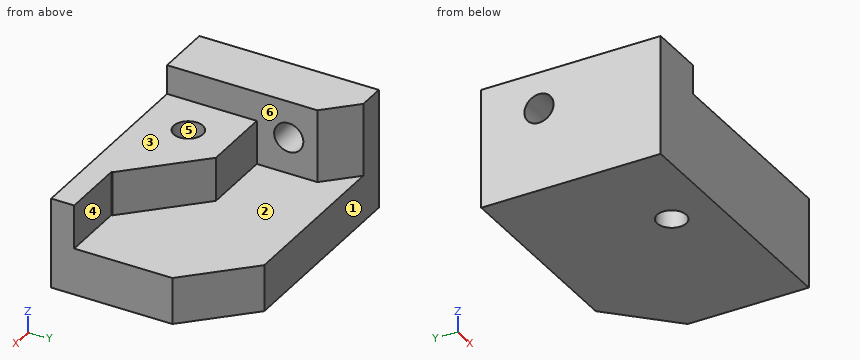
Autodesk Fusion 360 part; units mm, degrees
sketch "Sketch1" plane through (0, 0, 0) normal (0, 0, 1) x (1, 0, 0)
  line L0 (88.0885, 61.5355) -> (-88.0885, 61.5355)
  line L1 (-88.0885, 61.5355) -> (-88.0885, -61.5355)
  line L2 (-88.0885, -61.5355) -> (88.0885, -61.5355)
  line L3 (88.0885, -61.5355) -> (88.0885, 61.5355)
  line L4 (88.0885, 61.5355) -> (-88.0885, -61.5355) construction
  line L5 (-88.0885, 61.5355) -> (88.0885, -61.5355) construction
extrude "Extrude1" add sketch "Sketch1" along normal blind 32
chamfer "Chamfer1" distance 40 angle 45 1 edges at (88.0885, 61.5355, 16)
sketch "Sketch2" plane through (0, 0, 32) normal (0, 0, 1) x (-1, 0, 0)
  line L0 (-88.0885, -21.5355) -> (-48.0885, -61.5355)
  line L1 (-48.0885, -61.5355) -> (88.0885, -61.5355)
  line L2 (88.0885, -61.5355) -> (88.0885, 61.5355)
  line L3 (88.0885, 61.5355) -> (-88.0885, 61.5355)
  line L4 (-88.0885, 61.5355) -> (-88.0885, -21.5355)
  line L5 (88.0885, 61.5355) -> (49.7061, 61.5355)
  line L6 (49.7061, 61.5355) -> (49.7061, -61.5355)
  line L7 (49.7061, -61.5355) -> (88.0885, -61.5355)
  line L8 (88.0885, -61.5355) -> (88.0885, 61.5355)
extrude "Extrude2" add sketch "Sketch2" along normal blind 50 contours L1 L2 L3 L5 L6 L7 L8
sketch "Sketch3" plane through (0, 61.5355, 0) normal (0, 1, 0) x (-1, 0, 0)
  line L0 (-48.0885, 32) -> (-48.0885, 0)
  line L1 (-48.0885, 0) -> (88.0885, 0)
  line L2 (88.0885, 0) -> (88.0885, 82)
  line L3 (88.0885, 82) -> (49.7061, 82)
  line L4 (49.7061, 82) -> (49.7061, 32)
  line L5 (49.7061, 32) -> (-48.0885, 32)
chamfer "Chamfer2" distance 20 angle 45 1 edges at (-49.7061, 61.5355, 57)
sketch "Sketch4" plane through (0, 0, 32) normal (0, 0, 1) x (-1, 0, 0)
  line L0 (49.7061, -41.5355) -> (49.7061, 61.5355)
  line L1 (49.7061, 61.5355) -> (-88.0885, 61.5355)
  line L2 (-88.0885, 61.5355) -> (-88.0885, -21.5355)
  line L3 (-88.0885, -21.5355) -> (-48.0885, -61.5355)
  line L4 (-48.0885, -61.5355) -> (69.7061, -61.5355)
  line L5 (69.7061, -61.5355) -> (49.7061, -41.5355)
  line L6 (49.7061, 61.5355) -> (-43.9087, 61.5355)
  line L7 (-43.9087, 61.5355) -> (-43.9087, 0)
  line L8 (-43.9087, 0) -> (49.7061, 0)
  line L9 (49.7061, 0) -> (49.7061, 61.5355)
extrude "Extrude3" add sketch "Sketch4" along normal blind 30 contours L0 L1 L6 L7 L8 L9
chamfer "Chamfer3" distance 45 angle 45 1 edges at (43.9087, 0, 47)
sketch "Sketch5" plane through (0, 0, 32) normal (0, 0, 1) x (-1, 0, 0)
  line L0 (49.7061, 0) -> (1.0913, 0)
  line L1 (1.0913, 0) -> (-43.9087, 45)
  line L2 (-43.9087, 45) -> (-43.9087, 61.5355)
  line L3 (-43.9087, 61.5355) -> (-88.0885, 61.5355)
  line L4 (-88.0885, 61.5355) -> (-88.0885, -21.5355)
  line L5 (-88.0885, -21.5355) -> (-48.0885, -61.5355)
  line L6 (-48.0885, -61.5355) -> (69.7061, -61.5355)
  line L7 (69.7061, -61.5355) -> (49.7061, -41.5355)
  line L8 (49.7061, -41.5355) -> (49.7061, 0)
  line L9 (-43.9087, 61.5355) -> (-88.0885, 61.5355)
  line L10 (-88.0885, 61.5355) -> (-88.0885, 45.7382)
  line L11 (-88.0885, 45.7382) -> (-43.9087, 45.7382)
  line L12 (-43.9087, 45.7382) -> (-43.9087, 61.5355)
extrude "Extrude4" add sketch "Sketch5" along normal blind 30 contours L2 L3 L4 L9 L10 L11 L12
sketch "Sketch6" plane through (0, 0, 62) normal (0, 0, 1) x (-1, 0, 0)
  line L0 (-43.9087, 45) -> (1.0913, 0)
  line L1 (1.0913, 0) -> (49.7061, 0)
  line L2 (49.7061, 0) -> (49.7061, 61.5355)
  line L3 (49.7061, 61.5355) -> (-88.0885, 61.5355)
  line L4 (-88.0885, 61.5355) -> (-88.0885, 45.7382)
  line L5 (-88.0885, 45.7382) -> (-43.9087, 45.7382)
  line L6 (-43.9087, 45.7382) -> (-43.9087, 45)
hole "Hole1" at (-49.7061, 21.9099, 57.0062) direction (-1, 0, 0) diameter 20 depth 0.01 tip angle 0.01
hole "Hole2" at (-20.3371, -30.0422, 62) direction (0, 0, -1) diameter 20 depth 0.01
hole "Hole3" at (-20.3371, -30.0422, 61.99) direction (0, 0, -1) diameter 20 depth 80
The model under review builds one solid part; all positions refer to its coordinate system, in mm. Face numbers are marked on the shaded views. A direction names the side the tool comes from. Round coordinates to 2 decimals unless told otherwise and drop trailing zeros. Order: outer loops, then holes, each group sorted by start corner. A loop starts at its lowest first (then second) coordinate and runs counter-clockwise, first axis right, second up.
Item 1: Machinability: for the marked faces 1, 2 and 3, which of the approach directions +Z, -Z, +X, -X, +Y, -Y give a long, thin tool a straight path to every point of the face, cutting with its end or side? Answer none if there is none.
Working result:
face 1: +Z, -Z, +X, -X, +Y
face 2: +Z, +X, +Y
face 3: +Z, +X, +Y, -Y
Item 2: Add section A-A, the plane x = -23.5. State the section outline as (y, z) points, and give its area (3 significant figures).
Working result:
outline: (-61.54, 0) - (-39.53, 0) - (-39.53, 62) - (-61.54, 62) - close; (-20.56, 0) - (61.54, 0) - (61.54, 32) - (0, 32) - (0, 62) - (-20.56, 62) - close
area: 4,610 mm2
Item 3: Add section C-C, the plane y = -9. State the section outline as (x, z) points, and give its area (3 significant figures).
Working result:
outline: (-88.09, 0) - (88.09, 0) - (88.09, 32) - (7.91, 32) - (7.91, 62) - (-49.71, 62) - (-49.71, 82) - (-88.09, 82) - close
area: 9,290 mm2
Item 4: Draft analysis for pull direction Y (two halves, no side actions). For the marked faces 4, 5 and 6, state which applies: released by +Y, released by -Y, zero draft, split by the parting line, or undercut.
Working result:
face 4: released by +Y
face 5: undercut
face 6: zero draft
Item 5: For pin 1 (24 mm diameter, centred on x = 71, z = 45.5, fed in from +Y); pin 2 (10 mm diameter, centred on x = 1.5, z = 63.5, fed in from +Y); pin 3 (15 mm diameter, centred on y = -35, z = 64.5, fed in from +X); pin 4 (0.6 mm diameter, centred on y = -45.5, z = 44, fed in from +X), all flat-tipped, find the tip position at first contact; note any pin that passes through.
Working result:
pin 1: stops at y = -45.74
pin 2: stops at y = 0
pin 3: stops at x = 40.98
pin 4: stops at x = 88.09
Item 6: Add section D-D, the plane x = 76. State the section outline as (y, z) points, and give its area (3 significant figures).
Working result:
outline: (-61.54, 0) - (33.62, 0) - (33.62, 32) - (-45.74, 32) - (-45.74, 62) - (-61.54, 62) - close
area: 3,520 mm2
Item 7: Add section B-B, the plane z = 43.5. State the section outline as (x, y) points, and give its area (3 significant figures).
Working result:
outline: (-88.09, -61.54) - (88.09, -61.54) - (88.09, -45.74) - (43.91, -45.74) - (43.91, -45) - (-1.09, 0) - (-49.71, 0) - (-49.71, 41.54) - (-69.71, 61.54) - (-88.09, 61.54) - close; hole circle Ø20 at (-20.34, -30.04)
area: 9,660 mm2
Item 8: To check wall thickness, follow probe 1 along Z at (x, y) = (-23, 10); probe 2 along X at (y, z) = (-46.5, 70.5); probe 3 along X at (y, z) = (-37, 44.5). State the ranges of each line that lie inside material, in increasing order.
Working result:
probe 1: z = 0 to 32
probe 2: x = -88.09 to -49.71
probe 3: x = -88.09 to -27.52, -13.15 to 35.91
